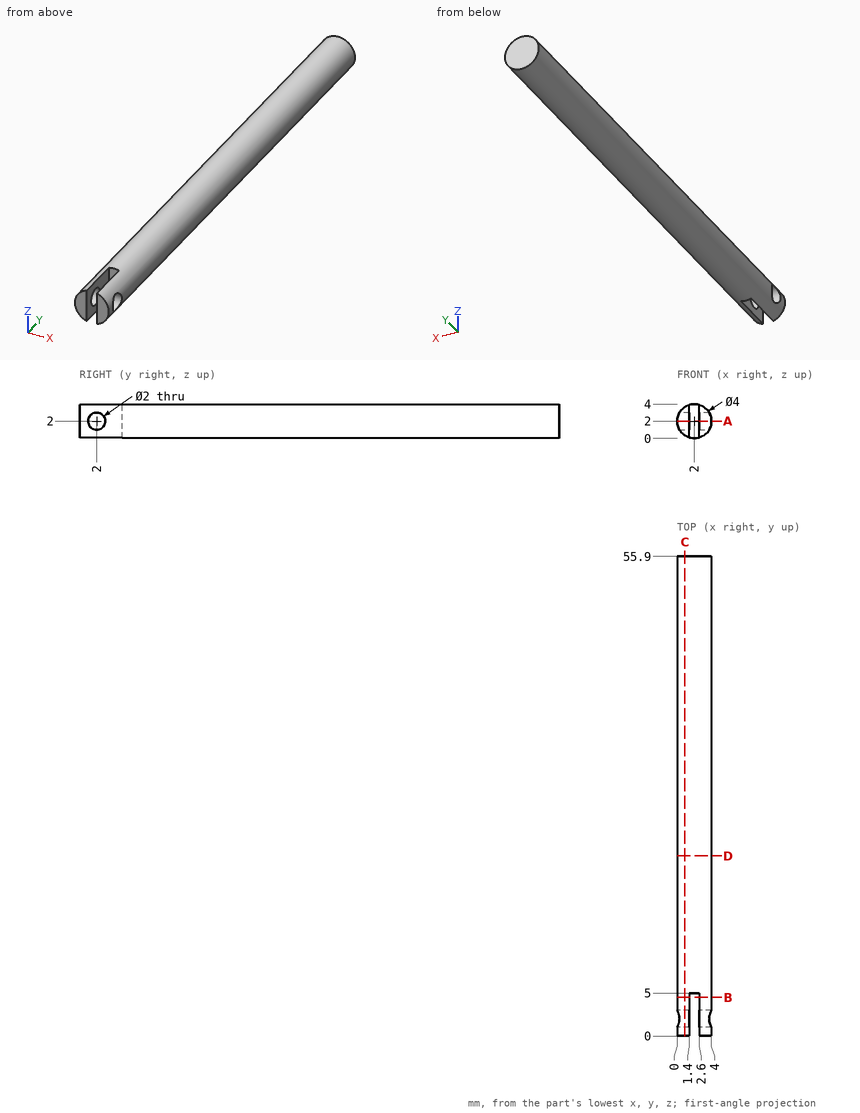
Design review of the part shown in the three views and the two pictorial views. Dimensions are in mm from the part's minimum x, y and z. Give positions to 0.01 mm unless a question says otherwise; leave off trailing zeros. Write each loop counter-clockwise with the first axis right and the second up, starting at its lowest first coordinate (ties: lowest second). Pieces come first, ordered by that corner, then holes. Notation, with made-up numbers: M 30.5,76 L 40.5,76 A25 cw 40.5,113 Z; hole C 4,5 d11. An arc over 180 degrees is marked long. One line per question, with ' | ' between items. Start each with the question number.
Item 1: Wall thickness on line 1 (Y direction, x = 0.9, z = 2); line 2 (X direction, y = 13, z = 1.9); line 3 (Y direction, x = 1.75, z = 1.9): over which ranges is each line inside the solid? List them lowest first. Write a range as from..to.
Item 2: We need section C-C on x = 0.9. Write out the cut boundary in (y, z), plus the area to 3 significant figures.
Item 3: We need section D-D on y = 21. Write out the cut boundary in (x, z), plus the area to 3 significant figures.
Item 4: We need section A-A on z = 2. Write out the cut boundary in (x, y).
Item 5: We need section B-B on y = 4.5. Write out the cut boundary in (x, z), plus the area to 3 significant figures.
Item 6: For pin 1 (1 mm diameter, centred on x = 3, y = 7.5, fed in from -Z); pin 2 (1.1 mm diameter, centred on y = 2, z = 1.5, fed in from +X), all flat-tipped, find the tip position at first contact; note any pin that passes through.
Results found:
1) line 1: y = 0..1, 3..55.9 | line 2: x = 0..4 | line 3: y = 5..55.9
2) outline: M 0,0.33 L 55.9,0.33 L 55.9,3.67 L 0,3.67 Z; hole C 2,2 d2 | area: 184 mm2
3) outline: C 2,2 d4 | area: 12.6 mm2
4) outline: M 0,0 L 1.4,0 L 1.4,1 L 0,1 Z; M 0,3 L 1.4,3 L 1.4,5 L 2.6,5 L 2.6,3 L 4,3 L 4,55.9 L 0,55.9 Z; M 2.6,0 L 4,0 L 4,1 L 2.6,1 Z
5) outline: M 1.4,0.09 L 1.4,3.91 A2 ccw Z; M 2.6,0.09 A2 ccw 2.6,3.91 Z | area: 7.84 mm2
6) pin 1: stops at z = 0.06 | pin 2: stops at x = 3.76
